Work out the finished part from the listing and answer in its coordinate system (mm). A direction names the side the tool comes from. Round coordinates to 2 decimals unless told otherwise and drop trailing zeros. Loops run counter-clockwise (first coordinate to the right, second up) from the corner with the lowest first, then second, coordinate; pieces in that order, holes last. Notation, with made-up numbers: (-14.5, 63) -> (10.5, 63) arc R26 cw to (10.5, 99) -> close; hole circle Ø7 at (31, -37). An arc over 180 degrees is marked (long way). Use one line per item in the form item = value.
```python
from build123d import *

# Parameters (mm, degrees)
SKETCH1_R           = 1.6
SKETCH1_R_2         = 1.1
SKETCH1_W           = 25
SKETCH1_H           = 15
BOSS_EXTRUDE1_DEPTH = 2
SKETCH2_R           = 1.6
CUT_EXTRUDE1_DEPTH  = 15
SKETCH3_R           = 1
CUT_EXTRUDE2_DEPTH  = 59.303758671


with BuildPart() as part:
    # Sketch1 → Boss-Extrude1 (new body)
    with BuildSketch(Plane(origin=(0, 0, 0), x_dir=(1, 0, 0), z_dir=(0, 1, 0))):
        Polygon((-20, 46.586782193), (20, 46.586782193), (35, 31.586782193), (35, 11.586782193), (25, 11.586782193), (25, -38.413217807), (35, -38.413217807), (29.754571716, -43.75543078), (-29.754571716, -43.75543078), (-35, -38.413217807), (-25, -38.413217807), (-25, 11.586782193), (-35, 11.586782193), (-35, 31.586782193), align=None)
        with Locations(Location((-30, 21.586782193, 0), (0, 0, 270))):
            Circle(SKETCH1_R, mode=Mode.SUBTRACT)
        with Locations(Location((30, 21.586782193, 0), (0, 0, 90))):
            Circle(SKETCH1_R, mode=Mode.SUBTRACT)
        with Locations(Location((0, 41.586782193, 0), (0, 0, 270))):
            Circle(SKETCH1_R, mode=Mode.SUBTRACT)
        with Locations(Location((-20, -4.413217807, 0), (0, 0, 270))):
            Circle(SKETCH1_R_2, mode=Mode.SUBTRACT)
        with Locations(Location((-20, -22.413217807, 0), (0, 0, 90))):
            Circle(SKETCH1_R_2, mode=Mode.SUBTRACT)
        with Locations(Location((20, -4.413217807, 0), (0, 0, 90))):
            Circle(SKETCH1_R_2, mode=Mode.SUBTRACT)
        with Locations(Location((20, -22.413217807, 0), (0, 0, 270))):
            Circle(SKETCH1_R_2, mode=Mode.SUBTRACT)
        with Locations(Location((-15, -37.75543078, 0), (0, 0, 270))):
            Circle(SKETCH1_R, mode=Mode.SUBTRACT)
        with Locations(Location((15, -37.75543078, 0), (0, 0, 90))):
            Circle(SKETCH1_R, mode=Mode.SUBTRACT)
        with Locations(Location((-15, 5.74456922, 0), (0, 0, 270))):
            Circle(SKETCH1_R, mode=Mode.SUBTRACT)
        with Locations(Location((15, 5.74456922, 0), (0, 0, 90))):
            Circle(SKETCH1_R, mode=Mode.SUBTRACT)
        with Locations(Location((-15, -30.25543078, 0), (0, 0, 270))):
            Circle(SKETCH1_R, mode=Mode.SUBTRACT)
        with Locations(Location((15, -30.25543078, 0), (0, 0, 90))):
            Circle(SKETCH1_R, mode=Mode.SUBTRACT)
        Polygon((12.330705785, 7.368716231), (17.905727496, 16.851286185), (11.871364798, 20.399027274), (6.296343087, 10.91645732), align=None, mode=Mode.SUBTRACT)
        with Locations((0, -13.413217807)):
            Rectangle(SKETCH1_W, SKETCH1_H, mode=Mode.SUBTRACT)
    extrude(amount=BOSS_EXTRUDE1_DEPTH)

    # Sketch2 → Cut-Extrude1 (cut)
    with BuildSketch(Plane(origin=(0, 2, 0), x_dir=(1, 0, 0), z_dir=(0, 1, 0))):
        with Locations(Location((-25, 27.900566449, 0), (0, 0, 270))):
            Circle(SKETCH2_R)
        with Locations(Location((25, 27.900566449, 0), (0, 0, 90))):
            Circle(SKETCH2_R)
    extrude(amount=-CUT_EXTRUDE1_DEPTH, mode=Mode.SUBTRACT)

    # Sketch3 → Cut-Extrude2 (cut, through all)
    with BuildSketch(Plane(origin=(0, 2, 0), x_dir=(1, 0, 0), z_dir=(0, 1, 0))):
        with Locations(Location((-7.5, 31.038288012, 0), (0, 0, 270))):
            Circle(SKETCH3_R)
        with Locations(Location((7.5, 31.038288012, 0), (0, 0, 90))):
            Circle(SKETCH3_R)
    extrude(amount=-CUT_EXTRUDE2_DEPTH, mode=Mode.SUBTRACT)


solid = part.part
```
(1) Find section C-C, the plane x = -7.5. Write down the section's boundary in (y, z).
Completed:
outline = (0, -46.59) -> (2, -46.59) -> (2, -32.04) -> (0, -32.04) -> close; (0, -30.04) -> (2, -30.04) -> (2, 5.91) -> (0, 5.91) -> close; (0, 20.91) -> (2, 20.91) -> (2, 43.76) -> (0, 43.76) -> close
(2) Find section D-D, the plane x = 15. Write down the section's boundary in (y, z).
Completed:
outline = (0, -46.59) -> (2, -46.59) -> (2, -18.56) -> (0, -18.56) -> close; (0, -11.91) -> (2, -11.91) -> (2, -7.34) -> (0, -7.34) -> close; (0, -4.14) -> (2, -4.14) -> (2, 28.66) -> (0, 28.66) -> close; (0, 31.86) -> (2, 31.86) -> (2, 36.16) -> (0, 36.16) -> close; (0, 39.36) -> (2, 39.36) -> (2, 43.76) -> (0, 43.76) -> close
(3) For faces 4 (the flat face through (27.395, 0.986, -39.192)), 5 (the flat face through (9.27, 0.99, -9.17)), 6 (the flat face through (-30, 1, -11.587)), determine the directions among +Z, -Z, +X, -X, +Y, -Y from which every point of the face is accessible in a straight line to the end or side of a thin tool.
Completed:
face_4 = -Z, +X, +Y, -Y
face_5 = +Y, -Y
face_6 = -X, +Y, -Y
(4) Find section B-B, the plane z = 16. Write down the section's boundary in (x, y), then the cut area to 3 significant figures.
Completed:
outline = (-25, 0) -> (-12.5, 0) -> (-12.5, 2) -> (-25, 2) -> close; (12.5, 0) -> (25, 0) -> (25, 2) -> (12.5, 2) -> close
area = 50.0 mm2
(5) Consider L1, parallel to X at y = 0.1, z = 39; L2, parallel to X at y = 1.1, z = -5.5; L3, parallel to X at y = 0.35, z = 6. Determine where each line is inside the solid, lowest interval first.
Completed:
L1 = -34.42 to -16.01, -13.99 to 13.99, 16.01 to 34.42
L2 = -25 to -16.58, -13.42 to 13.42, 16.58 to 25
L3 = -25 to -12.5, 12.5 to 25
(6) Given P1, Ø2.5, axis at x = -25, z = -27.9, coming from the +Y side; P2, Ø0.6, axis at x = 30.5, y = 1, coming from the +Z side; P3, Ø0.6, axis at y = 0.5, z = 13.5, coming from the +X side, each flat-ended and moving along its own axis, determine where each tip first touches the part or whether it passes through.
Completed:
P1 = through
P2 = 43.3
P3 = 25
(7) Find section A-A, the plane x = -15. Write down the section's boundary in (y, z), then the cut area to 3 significant figures.
Completed:
outline = (0, -46.59) -> (2, -46.59) -> (2, -7.34) -> (0, -7.34) -> close; (0, -4.14) -> (2, -4.14) -> (2, 28.66) -> (0, 28.66) -> close; (0, 31.86) -> (2, 31.86) -> (2, 36.16) -> (0, 36.16) -> close; (0, 39.36) -> (2, 39.36) -> (2, 43.76) -> (0, 43.76) -> close
area = 161 mm2
(8) For a pull along X with two mould halves and no side action, classify faces 1 (the flat face through (0, 1, 20.913)), 2 (the flat face through (30, 1, 38.413)), 3 (the flat face through (35, 1, -22)) as +X half, -X half, draft (parallel to the pull), parting line (faces both ways), or undercut.
Completed:
face_1 = undercut
face_2 = draft
face_3 = +X half
